Input: dimensioned drawing with shaded views. Units: mm. Origin: part minimum x, y, z. A direction names the side the tool comes from. Give positions to 0.01 mm unless a question says otherwise; leave off trailing zeros. Write each loop counter-clockwise with the first axis right and the second up, starting at its lowest first coordinate (ties: lowest second). Pieces come first, ordered by that corner, then holes. Notation, with made-up numbers: (5.5, 79) - (44.5, 79) arc R19 ccw to (44.5, 91) - close; hole circle Ø10 at (-27, 78). An arc over 180 degrees is marked (long way). Answer as CSV lines item,"result".
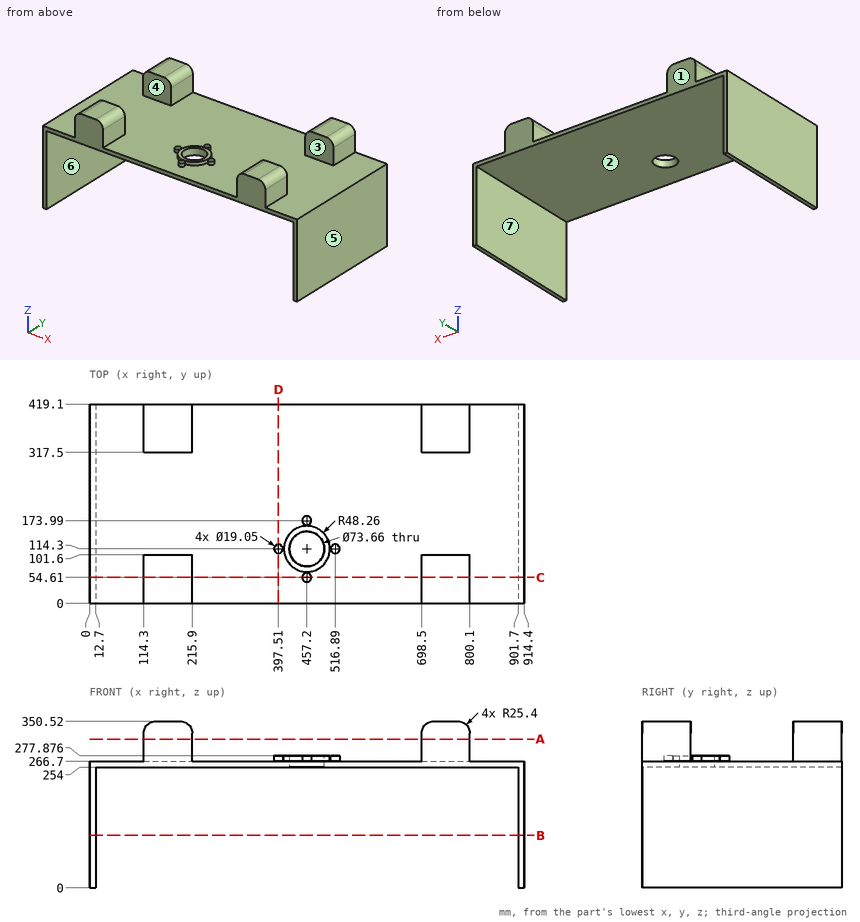
Item 1: Cut plane B-B on z = 110.5. Return the cut outline in (x, y), plus the area to 3 significant figures.
The answers:
outline,"(0, 0) - (12.7, 0) - (12.7, 419.1) - (0, 419.1) - close; (901.7, 0) - (914.4, 0) - (914.4, 419.1) - (901.7, 419.1) - close"
area,"10,600 mm²"
Item 2: Cut plane A-A on z = 313. Return the cut outline in (x, y).
The answers:
outline,"(114.3, 0) - (215.9, 0) - (215.9, 101.6) - (114.3, 101.6) - close; (114.3, 317.5) - (215.9, 317.5) - (215.9, 419.1) - (114.3, 419.1) - close; (698.5, 0) - (800.1, 0) - (800.1, 101.6) - (698.5, 101.6) - close; (698.5, 317.5) - (800.1, 317.5) - (800.1, 419.1) - (698.5, 419.1) - close"
Item 3: Contact query for flat-ended pins moving along their axis: pin 1 (4 mm diameter, centred on x = 583.5, y = 80, fed in from +Z); pin 2 (9.5 mm diameter, centred on x = 394.5, y = 115.5, fed in from +Z); pin 3 (5 mm diameter, centred on x = 607, y = 150, fed in from -Z). Output: stop coordinate, or through.
The answers:
pin 1,"z = 266.7"
pin 2,"z = 277.88"
pin 3,"z = 254"
Item 4: Reachability of the marked faces 1, 2 and 3 from +Z, -Z, +X, -X, +Y, -Y: full face, straight path, thin tool, end or side. Return the list, or none.
The answers:
face 1,"+Z, -Z, +X, -X, +Y"
face 2,"-Z, +Y, -Y"
face 3,"+Z, +X, -X"
Item 5: Ray query, line 1 (Y direction, x = 457.2, z = 266); line 2 (X direction, y = 371.5, z = 326.5); line 3 (X direction, y = 193.5, z = 72.5). Return the intervals inside material, ascending. Write a range as from..to.
The answers:
line 1,"0..77.47, 151.13..419.1"
line 2,"114.34..215.86, 698.54..800.06"
line 3,"0..12.7, 901.7..914.4"
Item 6: Mould query, pull axis X, two halves, no side actions, for the marked faces 4, 5, 6 and 7. Classes: +X half, -X half, draft (parallel to the pull), parting line (faces both ways), or undercut.
The answers:
face 4,"draft"
face 5,"+X half"
face 6,"undercut"
face 7,"undercut"
Item 7: Cut plane C-C on y = 54.61. Return the cut outline in (x, z) (3 decimals), plus the area to 3 significant figures.
The answers:
outline,"(0, 0) - (12.7, 0) - (12.7, 254) - (901.7, 254) - (901.7, 0) - (914.4, 0) - (914.4, 266.7) - (800.1, 266.7) - (800.1, 325.12) arc R25.4 ccw to (774.7, 350.52) - (723.9, 350.52) arc R25.4 ccw to (698.5, 325.12) - (698.5, 266.7) - (466.725, 266.7) - (466.725, 277.876) - (447.675, 277.876) - (447.675, 266.7) - (215.9, 266.7) - (215.9, 325.12) arc R25.4 ccw to (190.5, 350.52) - (139.7, 350.52) arc R25.4 ccw to (114.3, 325.12) - (114.3, 266.7) - (0, 266.7) - close"
area,"34,800 mm²"
Item 8: Cut plane D-D on x = 397.51. Return the cut outline in (y, z) (3 decimals), plus the area to 3 significant figures.
The answers:
outline,"(0, 254) - (419.1, 254) - (419.1, 266.7) - (123.825, 266.7) - (123.825, 277.876) - (104.775, 277.876) - (104.775, 266.7) - (0, 266.7) - close"
area,"5,540 mm²"
